Input: part model. Units: mm. Frame: model coordinates. Face numbers are marked on the shaded views. A direction names the side the tool comes from. Coordinates: 2 decimals unless noted, no trailing zeros. Order: outer loops, then holes, each group sorted by start corner. A loop starts at its lowest first (then second) coordinate and runs counter-clockwise, first axis right, second up.
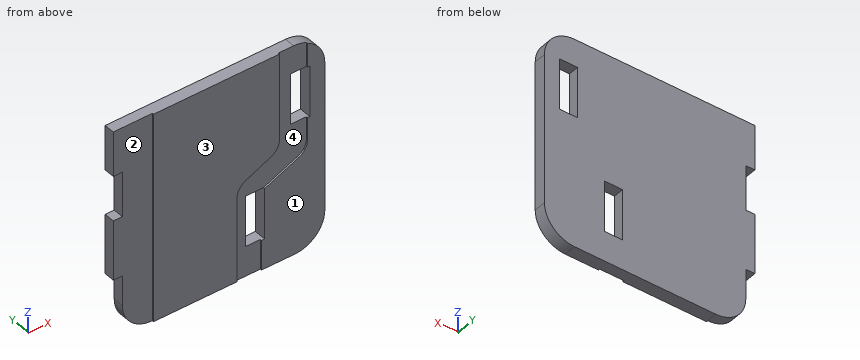
from build123d import *

# Parameters (mm, degrees)
SKETCH1_W           = 0.6
SKETCH1_H           = 1.7
BOSS_EXTRUDE1_DEPTH = 0.4
FILLET1_R           = 1
SKETCH2_W           = 1.728090014
SKETCH2_H           = 7
CUT_EXTRUDE1_DEPTH  = 0.05


with BuildPart() as part:
    # Sketch1 → Boss-Extrude1 (new body)
    with BuildSketch(Plane(origin=(0, 0, 0), x_dir=(1, 0, 0), z_dir=(0, 1, 0))):
        Polygon((0, 0), (7, 0), (7, 7), (0.3, 7), (0.3, 5), (0, 5), (0, 3), (0.3, 3), (0.3, 1.5), (0, 1.5), align=None)
        with Locations((4.7, 5.15)):
            Rectangle(SKETCH1_W, SKETCH1_H, mode=Mode.SUBTRACT)
        with Locations((6.2, 1.75)):
            Rectangle(SKETCH1_W, SKETCH1_H, mode=Mode.SUBTRACT)
    extrude(amount=BOSS_EXTRUDE1_DEPTH)

    # Fillet1
    fillet1_edges = [part.edges().sort_by_distance(p)[0] for p in [
        (0.3, 0.2, -7),
        (7, 0.2, -7),
        (7, 0.2, 0),
    ]]
    fillet(fillet1_edges, radius=FILLET1_R)

    # Sketch2 → Cut-Extrude1 (cut)
    with BuildSketch(Plane.XZ):
        with BuildLine():
            Line((5, -6), (4.891522781, -6))
            Line((4.891522781, -6), (4.891522781, -7.295431915))
            Line((4.891522781, -7.295431915), (4.07762411, -7.295431915))
            Line((4.07762411, -7.295431915), (4.07762411, -4.178910814))
            ThreePointArc((4.07762411, -4.178910814), (4.156244956, -3.909764741), (4.367382545, -3.725260636))
            Line((4.367382545, -3.725260636), (5.20570378, -3.336745481))
            ThreePointArc((5.20570378, -3.336745481), (5.416841369, -3.152241376), (5.495462215, -2.883095303))
            Line((5.495462215, -2.883095303), (5.495462215, 0.578390888))
            Line((5.495462215, 0.578390888), (6.425754314, 0.578390888))
            Line((6.425754314, 0.578390888), (6.425754314, -0.9))
            Line((6.425754314, -0.9), (6.5, -0.9))
            Line((6.5, -0.9), (6.5, -2.6))
            Line((6.5, -2.6), (6.425754314, -2.6))
            Line((6.425754314, -2.6), (6.425754314, -3.345351228))
            ThreePointArc((6.425754314, -3.345351228), (6.344600523, -3.618422378), (6.127482902, -3.802850492))
            Line((6.127482902, -3.802850492), (5, -4.3))
            Line((5, -4.3), (5, -6))
        make_face()
        with Locations((0.435954993, -3.5)):
            Rectangle(SKETCH2_W, SKETCH2_H)
    extrude(amount=-CUT_EXTRUDE1_DEPTH, mode=Mode.SUBTRACT)


solid = part.part
Item 1: Draft query along X for the marked faces 3 and 4. Return one class per face: pulls with the +X half, pulls with the -X half, needs draft (parallel to the pull), parting line crosses it, or undercut.
Response values:
face 3: needs draft
face 4: undercut
Item 2: Cut plane A-A on z = -2.25. Return loops of the section in (x, y), then the cut area to 3 significant figures.
Response values:
outline: (0.3, 0.05) - (1.3, 0.05) - (1.3, 0) - (5.5, 0) - (5.5, 0.05) - (5.9, 0.05) - (5.9, 0.4) - (0.3, 0.4) - close; (6.5, 0) - (7, 0) - (7, 0.4) - (6.5, 0.4) - close
area: 2.37 mm2
Item 3: Access query for the marked faces 1 and 2. Directions: +Z, -Z, +X, -X, +Y, -Y. A direction counts if a zero-diameter tool reaches every point of the face in a straight line with its end or side. Return the directions, or none.
Response values:
face 1: +Z, -Z, +X, -X, -Y
face 2: +Z, -Z, -X, -Y
Item 4: Ray query, probe 1 along X at (y, z) = (0.35, -5.5); probe 2 along Z at (x, y) = (6, 0.1); probe 3 along X at (y, z) = (0.15, -4.5). Return the intervals inside material, ascending.
Response values:
probe 1: x = 0.3 to 4.4, 5 to 7
probe 2: z = -7 to -2.6, -0.9 to 0
probe 3: x = 0 to 4.4, 5 to 7
Item 5: Cut plane C-C on x = 4.75. Return loops of the section in (y, z), then the cut area to 3 significant figures.
Response values:
outline: (0, -3.55) - (0.05, -3.55) - (0.05, -4.3) - (0.4, -4.3) - (0.4, 0) - (0, 0) - close; (0.05, -7) - (0.4, -7) - (0.4, -6) - (0.05, -6) - close
area: 2.03 mm2
Item 6: Cut plane D-D on z = -6.25. Return loops of the section in (x, y), then the cut area to 3 significant figures.
Response values:
outline: (0.33, 0.05) - (1.3, 0.05) - (1.3, 0) - (4.08, 0) - (4.08, 0.05) - (4.89, 0.05) - (4.89, 0) - (6.97, 0) - (6.97, 0.4) - (0.33, 0.4) - close
area: 2.57 mm2
Item 7: Cut plane B-B on y = 0.2. Return loops of the section in (x, z).
Response values:
outline: (0, -5) - (0.3, -5) - (0.3, -6) arc R1 ccw to (1.3, -7) - (6, -7) arc R1 ccw to (7, -6) - (7, -1) arc R1 ccw to (6, 0) - (0, 0) - (0, -1.5) - (0.3, -1.5) - (0.3, -3) - (0, -3) - close; hole (4.4, -6) - (5, -6) - (5, -4.3) - (4.4, -4.3) - close; hole (5.9, -2.6) - (6.5, -2.6) - (6.5, -0.9) - (5.9, -0.9) - close
